Verification items for this drawing (mm, ordinates from the low corner). A direction names the side the tool comes from. Give positions to 0.01 mm unless a question says otherwise; leave off trailing zeros. Loops run counter-clockwise (first coordinate to the right, second up) from the corner with the lowest first, then second, coordinate; pieces in that order, holes last. Notation, with made-up numbers: (-38.75, 67.5) -> (4.25, 67.5) arc R32 cw to (4.25, 96.5) -> close; hole circle Ø2 at (31.5, -36). An arc over 180 degrees is marked (long way). Write item = value, one per line.
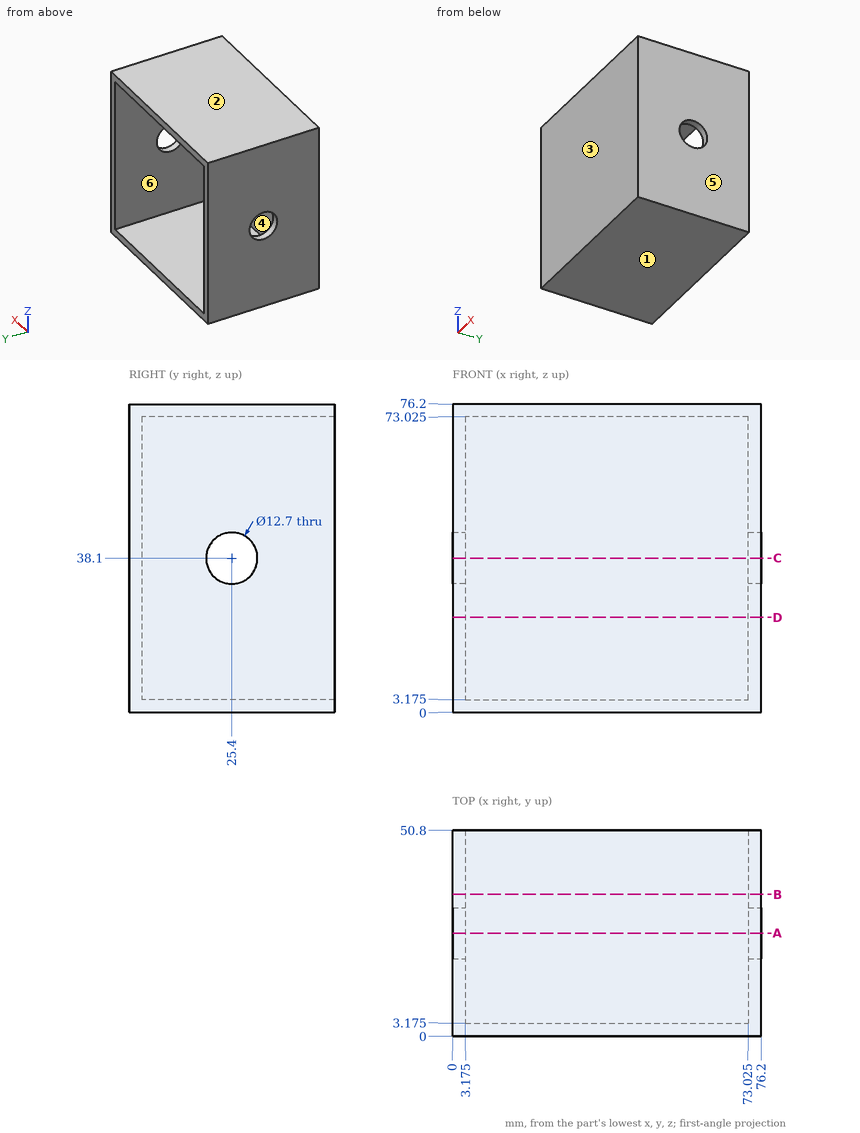
Item 1: Section check B-B, the plane y = 35. Record the cut outline in (x, z) (3 decimals), plus the area to 3 significant figures.
Answer:
outline = (0, 0) -> (76.2, 0) -> (76.2, 76.2) -> (0, 76.2) -> close; hole (3.175, 3.175) -> (73.025, 3.175) -> (73.025, 73.025) -> (3.175, 73.025) -> close
area = 927 mm^2
Item 2: Section check A-A, the plane y = 25.4. Record the cut outline in (x, z) (3 decimals).
Answer:
outline = (0, 0) -> (76.2, 0) -> (76.2, 31.75) -> (73.025, 31.75) -> (73.025, 3.175) -> (3.175, 3.175) -> (3.175, 31.75) -> (0, 31.75) -> close; (0, 44.45) -> (3.175, 44.45) -> (3.175, 73.025) -> (73.025, 73.025) -> (73.025, 44.45) -> (76.2, 44.45) -> (76.2, 76.2) -> (0, 76.2) -> close
Item 3: Section check D-D, the plane z = 23.5. Record the cut outline in (x, y) (3 decimals).
Answer:
outline = (0, 0) -> (76.2, 0) -> (76.2, 50.8) -> (73.025, 50.8) -> (73.025, 3.175) -> (3.175, 3.175) -> (3.175, 50.8) -> (0, 50.8) -> close
Item 4: Draft check along Z on the marked faces 1, 2, 3 and 4. Enter one of: +Z half, -Z half, draft (parallel to the pull), parting line (faces both ways), or undercut.
Answer:
face_1 = -Z half
face_2 = +Z half
face_3 = draft
face_4 = undercut
Item 5: Tool access check on the marked faces 5 and 6. Record the directions out of +Z, -Z, +X, -X, +Y, -Y that give a thin tool (end or side, any length) a straight path to the whole face; none if there is none.
Answer:
face_5 = +Z, -Z, +X, +Y, -Y
face_6 = +Y
Item 6: Section check C-C, the plane z = 38.1. Record the cut outline in (x, y) (3 decimals), plus the area to 3 significant figures.
Answer:
outline = (0, 0) -> (76.2, 0) -> (76.2, 19.05) -> (73.025, 19.05) -> (73.025, 3.175) -> (3.175, 3.175) -> (3.175, 19.05) -> (0, 19.05) -> close; (0, 31.75) -> (3.175, 31.75) -> (3.175, 50.8) -> (0, 50.8) -> close; (73.025, 31.75) -> (76.2, 31.75) -> (76.2, 50.8) -> (73.025, 50.8) -> close
area = 464 mm^2
Item 7: Thickness scan on L1, parallel to X at y = 43, z = 42 (3 decimals); L2, parallel to Z at x = 74, y = 25. Record the ranges inside material, lowest first. Write a range as [from, to].
Answer:
L1 = [0, 3.175], [73.025, 76.2]
L2 = [0, 31.76], [44.44, 76.2]
Item 8: Gauge pin test, flat ends, axial feed: pin 1 (24 mm diameter, centred on x = 50, y = 38.5, fed in from -Z); pin 2 (21 mm diameter, centred on x = 27, z = 38.5, fed in from +Y) (3 decimals). Record the tip position at first contact, or that the pin passes through.
Answer:
pin_1 = 0
pin_2 = 3.175
